Here's how the part is built. I have some questions about the finished solid (model axes, mm). Face numbers are marked on the shaded views. A direction names the side the tool comes from. Coordinates: 2 decimals unless noted, no trailing zeros. Loops run counter-clockwise (first coordinate to the right, second up) from the corner with the lowest first, then second, coordinate; pieces in that order, holes last. Notation, with made-up numbers: M -29.5,76 L -10.5,76 A14 ccw -10.5,102 Z; hole C -4,73.25 d1. An arc over 180 degrees is marked long. Use one line per item in the form item = value. Start each with the question number.
(1) Thinking about a two-plate mould opening in X: for the marked faces 6, 7 and 8, which applies, +X half, -X half, draft (parallel to the pull), parting line (faces both ways), or undercut?
(2) Will these pins go through, and if not, where does the flat tip stop? P1, Ø14, axis at x = -1.5, y = 403.5, coming from the +Z side; P2, Ø10, axis at x = 2, z = -31, coming from the +Y side; P3, Ø3, axis at x = -25.5, y = 143, coming from the +Z side; P4, Ø3, axis at x = -43.5, z = 12.5, coming from the -Y side.
(3) Imagine slicing it at A-A, the plane y = 198. Please give me the cut outline in (x, z).
(4) Please list where these lines run through material, in increasing order: L1, parallel to Z at x = 0, y = 337; L2, parallel to Y at x = 30, z = 37; L3, parallel to Y at x = -48.5, z = -15 (3 decimals).
(5) Imagine slicing it at B-B, the plane x = 0. State how many separate pieces and enclosed holes the cut face has, and give its area (3 significant figures).
(6) On a 3-axis mill with a long thin cutter (end or side, diameter ignored), from which of +Z, -Z, +X, -X, +Y, -Y can I reach the whole of each face in a straight line? I mean the marked faces 1, 2, 3, 4 and 5. Say none if no direction works.
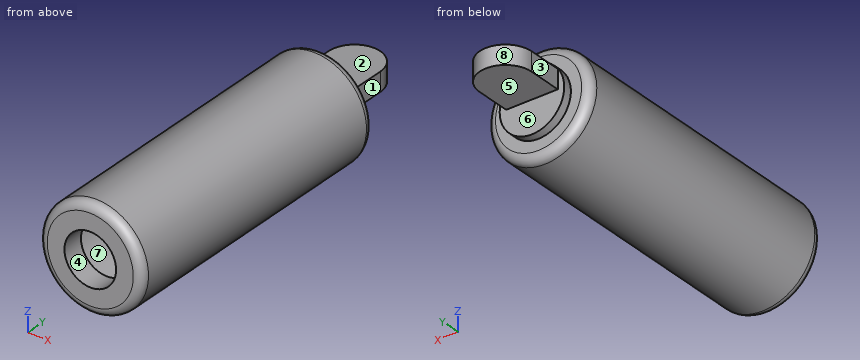
Autodesk Inventor part; units mm, degrees
ref_plane "Work Plane1" through (0, 175, 0) normal (0, -1, 0) x (1, 0, 0)
ref_plane "YZ Plane" through (0, 0, 0) normal (1, 0, 0) x (0, 1, 0)
ref_plane "XZ Plane" through (0, 0, 0) normal (0, 1, 0) x (-1, 0, 0)
sketch "Sketch1" plane through (0, 0, 0) normal (0, 1, 0) x (-1, 0, 0)
  circle A0 centre (0, 0) radius 60
  circle A1 centre (0, 0) radius 30
  dimension "d0" = 120
  dimension "d3" = 60
extrude "Extrusion1" add sketch "Sketch1" along normal blind 350
sketch "Sketch2" plane through (0, 350, 0) normal (0, 1, 0) x (1, 0, 0)
  circle A0 centre (0, 0) radius 37.5
  dimension "d7" = 75
extrude "Extrusion2" add sketch "Sketch2" along normal blind 10
sketch "Sketch4" plane through (0, 360, 0) normal (0, 1, 0) x (1, 0, 0)
  point P0 (0, 0)
sketch "Sketch5" plane through (0, 0, 0) normal (0, 0, 1) x (1, 0, 0)
  line L0 (37.5, 360) -> (-37.5, 360)
  line L1 (0, 360) -> (0, 400)
  circle A0 centre (0, 400) radius 30
  line L2 (30, 400) -> (30, 360)
  line L3 (-30, 400) -> (-30, 360)
  line L4 (-30, 360) -> (30, 360)
  point P0 (0, 0)
  dimension "d13" = 40
  dimension "d14" = 60
extrude "Extrusion4" add sketch "Sketch5" along normal blind 22
fillet "Fillet1" radius 10 2 edges at (60, 350, 0) (60, 0, 0)
ref_plane "Work Plane1" through (0, 175, 0) normal (0, -1, 0) x (1, 0, 0)
sketch "Sketch6" plane through (0, 175, 0) normal (0, -1, 0) x (1, 0, 0)
  circle A0 centre (0, 0) radius 57.5
  dimension "d23" = 115
extrude "Extrusion5" cut sketch "Sketch6" along normal mid plane 300
shell "Shell1" thickness 6.5 removed faces 0
properties part number "Arm1" material "Aluminum 6061"
Answer:
q1.face_6 = draft
q1.face_7 = undercut
q1.face_8 = parting line
q2.P1 = 22
q2.P2 = 360
q2.P3 = 54.99
q2.P4 = 0
q3.outline = C 0,0 d120; hole C 0,0 d115
q4.L1 = -60 to -53.5, -36.5 to -30, 30 to 36.5, 53.5 to 60
q4.L2 = 0 to 6.5, 18.5 to 25, 325 to 331.5, 343.5 to 350
q4.L3 = 0.029 to 6.585, 18.5 to 25, 325 to 331.5, 343.415 to 349.971
q5.separate_pieces = 1
q5.enclosed_holes = 5
q5.area = 5,300 mm²
q6.face_1 = +Z, -Z, +X, +Y
q6.face_2 = +Z, +X, -X, +Y
q6.face_3 = +Z, -Z, -X, +Y
q6.face_4 = -Y
q6.face_5 = -Z, +X, -X, +Y
